from build123d import *

# Parameters (mm, degrees)
SKETCH3_W         = 0.6858
SKETCH3_H         = 3.048
SKETCH4_W         = 0.3429
SKETCH4_H         = 0.3429
CIRPATTERN1_COUNT = 2
CIRPATTERN1_ANGLE = 90


with BuildPart() as part:
    # BodySke → Base-Revolve (revolve)
    with BuildSketch(Plane.XY):
        Polygon((0, 0), (0, 1.8669), (0.404209595, 1.8669), (1.2954, 1.0922), (6.35, 1.0922), (6.35, 0), align=None)
    revolve(axis=Axis((-6.35, 0, 0), (1, 0, 0)))

    # Sketch3 → Cross section 0
    with BuildSketch(Plane.ZY):
        Rectangle(SKETCH3_W, SKETCH3_H)
    # Sketch4 → Cross section 1
    with BuildSketch(Plane.ZY.offset(-1.6764)):
        Rectangle(SKETCH4_W, SKETCH4_H)
    cross = loft(mode=Mode.SUBTRACT)

    # CirPattern1: Cross ×2 about axis
    cirpattern1_axis = Axis((0, 0, 0), (1, 0, 0))
    for i in range(1, CIRPATTERN1_COUNT):
        add(cross.rotate(cirpattern1_axis, i * CIRPATTERN1_ANGLE / (CIRPATTERN1_COUNT - 1)), mode=Mode.SUBTRACT)


solid = part.part
Check sheet for the modelled part. Datum: model origin and axes. Units: mm. A direction names the side the tool comes from. Coordinates: 2 decimals unless noted, no trailing zeros. Loops run counter-clockwise (first coordinate to the right, second up) from the corner with the lowest first, then second, coordinate; pieces in that order, holes last. Notation, with made-up numbers: (41.25, 64) -> (86.25, 64) arc R17 cw to (86.25, 92) -> close; hole circle Ø8 at (48, 68.5). An arc over 180 degrees is marked (long way). Answer in a Markdown table with one row per item.
1. Go/stop test with flat-tipped pins: pin 1 (1.5 mm diameter, centred on x = 4.5, y = 0.5, fed in from +Z); pin 2 (1 mm diameter, centred on x = 4.5, y = -1, fed in from -Z); pin 3 (1 mm diameter, centred on x = 1, z = 0.5, fed in from +Y). Record where each tip stops, or that it passes through.
Check values:
| item | result |
|---|---|
| pin 1 | stops at z = 1.09 |
| pin 2 | stops at z = -0.97 |
| pin 3 | stops at y = 1.73 |
2. Material ranges on line 1 along Y through (x, z) = (1.25, 0.3); line 2 along Y through (x, z) = (1.75, 0.9); line 3 along Y through (x, z) = (1.75, -0.5), recorded low to high. Write a range as [from, to].
Check values:
| item | result |
|---|---|
| line 1 | y = [-1.09, -0.22], [0.22, 1.09] |
| line 2 | y = [-0.62, 0.62] |
| line 3 | y = [-0.97, 0.97] |
3. Sectioned sample at A-A, the plane x = 5.75. Record the boundary of the cut face in (y, z), then the cut area to 3 significant figures.
Check values:
| item | result |
|---|---|
| outline | circle Ø2.18 at (0, 0) |
| area | 3.75 mm2 |
4. Access from +Z, -Z, +X, -X, +Y, -Y to the whole of each face (thin tool, end or side, straight path). Record for faces 1 (the face through (6.35, 0, 0)), 2 (the face through (3.86, 1.04, 0.33)).
Check values:
| item | result |
|---|---|
| face 1 | +Z, -Z, +X, +Y, -Y |
| face 2 | +X |
